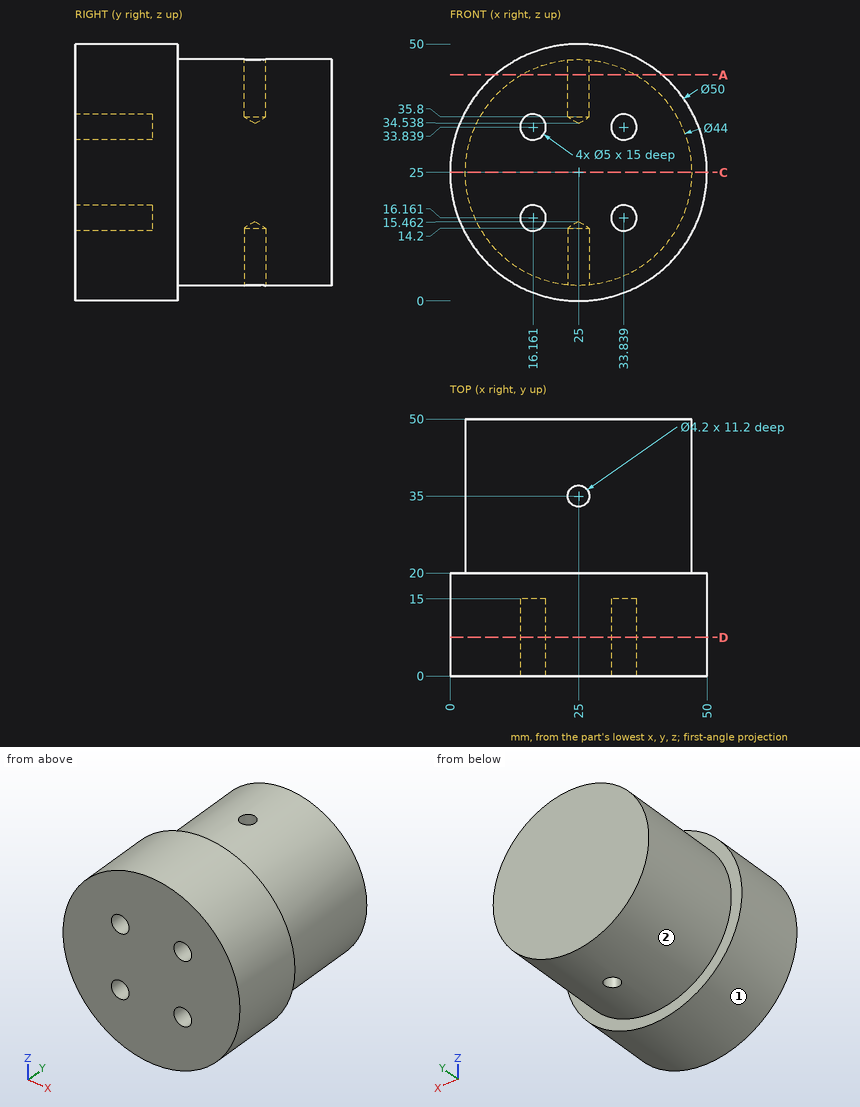
Geometry: see drawing. Coordinates: mm, zero at the bounding-box minimum. A direction names the side the tool comes from. Coordinates: 2 decimals unless noted, no trailing zeros. Order: outer loops, then holes, each group sorted by start corner. A loop starts at its lowest first (then second) coordinate and runs counter-clockwise, first axis right, second up. Notation, with made-up numbers: (19, -12.75) -> (68, -12.75) arc R20 ccw to (68, 9.25) -> close; hole circle Ø7 at (52.5, 0). An arc over 180 degrees is marked (long way). Write each question's results on one line, items separated by ' | '. Start each with the question number.
1) Material intervals for line 1 along Y through (x, z) = (25, 41); line 2 along Y through (x, z) = (29, 3); line 3 along X through (y, z) = (32, 25), sorted ascending.
2) First-contact query: pin 1 (2.5 mm diameter, centred on x = 33.5, z = 34, fed in from -Y); pin 2 (8 mm diameter, centred on y = 13.5, z = 34, fed in from +X) (3 decimals); pin 3 (4 mm diameter, centred on x = 25, y = 35, fed in from -Z). Flat tips, straight axial feed; report the tip coordinate or a pass-through.
3) Set-up query: the marked faces 1 and 2. Return all of +Z, -Z, +X, -X, +Y, -Y with unobstructed straight access to the full face (end or side cutting, diameter ignored); none if empty.
4) Cut plane A-A, the plane z = 44. Output: boundary loops of the cut face in (x, y), and give its area (3 significant figures).
5) Cut plane C-C, the plane z = 25. Output: boundary loops of the cut face in (x, y), and give its area (3 significant figures).
6) Cut plane D-D, the plane y = 7.5. Output: boundary loops of the cut face in (x, z).
Checks:
1) line 1: 0 to 32.9, 37.1 to 50 | line 2: 0 to 20 | line 3: 3 to 47
2) pin 1: y = 15 | pin 2: x = 49.495 | pin 3: z = 14.26
3) face 1: +Y, -Y | face 2: +Y
4) outline: (8.75, 0) -> (41.25, 0) -> (41.25, 20) -> (36.09, 20) -> (36.09, 50) -> (13.91, 50) -> (13.91, 20) -> (8.75, 20) -> close; hole circle Ø4.2 at (25, 35) | area: 1,300 mm^2
5) outline: (0, 0) -> (50, 0) -> (50, 20) -> (47, 20) -> (47, 50) -> (3, 50) -> (3, 20) -> (0, 20) -> close | area: 2,320 mm^2
6) outline: circle Ø50 at (25, 25); hole circle Ø5 at (16.16, 16.16); hole circle Ø5 at (16.16, 33.84); hole circle Ø5 at (33.84, 16.16); hole circle Ø5 at (33.84, 33.84)
